from build123d import *

# Parameters (mm, degrees)
F_01_START                                = -2
S01_GROUND_GUIDE_BORE_AND_BODY_R          = 6
S01_GROUND_GUIDE_BORE_AND_BODY_R_2        = 4.22
F_01_GROUND_GUIDE_BORE_AND_BODY_DEPTH     = 14
F_02_START                                = 12
S02_OUTBOARD_FLANGE_R                     = 7.65
S02_OUTBOARD_FLANGE_R_2                   = 4.22
F_02_OUTBOARD_FLANGE_DEPTH                = 1
F_03_START                                = -1.05
S03_EXTERNAL_RETAINING_RING_GROOVE_R      = 6.1
S03_EXTERNAL_RETAINING_RING_GROOVE_R_2    = 5.6
F_03_EXTERNAL_RETAINING_RING_GROOVE_DEPTH = 0.85


with BuildPart() as part:
    # S01 - Ground guide bore and body → 01 - Ground guide bore and body (new body)
    with BuildSketch(Plane.XY.offset(F_01_START)):
        Circle(S01_GROUND_GUIDE_BORE_AND_BODY_R)
        Circle(S01_GROUND_GUIDE_BORE_AND_BODY_R_2, mode=Mode.SUBTRACT)
    extrude(amount=F_01_GROUND_GUIDE_BORE_AND_BODY_DEPTH)

    # S02 - Outboard flange → 02 - Outboard flange (add)
    with BuildSketch(Plane.XY.offset(F_02_START)):
        Circle(S02_OUTBOARD_FLANGE_R)
        Circle(S02_OUTBOARD_FLANGE_R_2, mode=Mode.SUBTRACT)
    extrude(amount=F_02_OUTBOARD_FLANGE_DEPTH)

    # S03 - External retaining ring groove → 03 - External retaining ring groove (cut)
    with BuildSketch(Plane.XY.offset(F_03_START)):
        Circle(S03_EXTERNAL_RETAINING_RING_GROOVE_R)
        Circle(S03_EXTERNAL_RETAINING_RING_GROOVE_R_2, mode=Mode.SUBTRACT)
    extrude(amount=F_03_EXTERNAL_RETAINING_RING_GROOVE_DEPTH, mode=Mode.SUBTRACT)


solid = part.part
Geometry: final body of the model. Coordinates: model frame, mm. A direction names the side the tool comes from. Coordinates: 2 decimals unless noted, no trailing zeros. Order: outer loops, then holes, each group sorted by start corner. A loop starts at its lowest first (then second) coordinate and runs counter-clockwise, first axis right, second up.
1) Section A-A (x = 0). Return loops of the section in (y, z).
Result sheet:
outline: (-7.65, 12) - (-6, 12) - (-6, -0.2) - (-5.6, -0.2) - (-5.6, -1.05) - (-6, -1.05) - (-6, -2) - (-4.22, -2) - (-4.22, 13) - (-7.65, 13) - close; (4.22, -2) - (6, -2) - (6, -1.05) - (5.6, -1.05) - (5.6, -0.2) - (6, -0.2) - (6, 12) - (7.65, 12) - (7.65, 13) - (4.22, 13) - close
2) Set-up query: faces 5 (the cylindrical face through (-5.994, 0.264, -1.532)), 6 (the cylindrical face through (-1.658, -7.468, 12.493)), 7 (the flat face through (-5, 3, -1.05)). Return all of +Z, -Z, +X, -X, +Y, -Y with unobstructed straight access to the full face (end or side cutting, diameter ignored); none if empty.
Result sheet:
face 5: -Z
face 6: +Z, -Z
face 7: none
3) Section D-D (z = 7). Return loops of the section in (x, y), then the cut area to 3 significant figures.
Result sheet:
outline: circle Ø12 at (0, 0); hole circle Ø8.44 at (0, 0)
area: 57.2 mm2
4) Draft query along Z for faces 1 (the flat face through (-5, 3, -0.2)), 2 (the cylindrical face through (-6, 0, 6)), 3 (the flat face through (3.3, -3.3, 13)), 4 (the flat face through (-5, -4, 12)). Return one class per face: released by +Z, released by -Z, zero draft, split by the parting line, or undercut.
Result sheet:
face 1: undercut
face 2: zero draft
face 3: released by +Z
face 4: released by -Z
5) Ray query, probe 1 along Z at (x, y) = (-4, -4); probe 2 along Y at (x, z) = (0, 6); probe 3 along Z at (x, y) = (4, -6). Return the intervals inside material, ascending.
Result sheet:
probe 1: z = -2 to -1.05, -0.2 to 13
probe 2: y = -6 to -4.22, 4.22 to 6
probe 3: z = 12 to 13
6) Section C-C (y = -4.75). Return loops of the section in (x, z), then the cut area to 3 significant figures.
Result sheet:
outline: (-6, 12) - (-3.67, 12) - (-3.67, -0.2) - (-2.97, -0.2) - (-2.97, -1.05) - (-3.67, -1.05) - (-3.67, -2) - (3.67, -2) - (3.67, -1.05) - (2.97, -1.05) - (2.97, -0.2) - (3.67, -0.2) - (3.67, 12) - (6, 12) - (6, 13) - (-6, 13) - close
area: 113 mm2
7) First-contact query: P1, Ø3, axis at x = 5, z = -0.5, coming from the +Y side; P2, Ø4, axis at x = -0.5, y = 0.5, coming from the -Z side; P3, Ø2, axis at x = 4, z = 4, coming from the +Y side; P4, Ø4, axis at x = -5.5, z = 7, coming from the -Y side. Flat tips, straight axial feed; report the tip coordinate or a pass-through.
Result sheet:
P1: stops at y = 4.85
P2: passes through
P3: stops at y = 5.2
P4: stops at y = -4.87
